from build123d import *

# Parameters (mm, degrees)
EXTRUDE_1_DEPTH     = 3
SKETCH_2_R          = 1.7
SKETCH_2_R_2        = 1.57
CUT_EXTRUDE_1_DEPTH = 3
SKETCH_3_W          = 60
SKETCH_3_H          = 3
EXTRUDE_2_DEPTH     = 5
SKETCH_6_W          = 155
SKETCH_6_H          = 3
EXTRUDE_3_DEPTH     = 4
SKETCH_7_W          = 155
SKETCH_7_H          = 3
EXTRUDE_4_DEPTH     = 4
FILLET_1_R          = 10
CUT_EXTRUDE_3_DEPTH = 4
FILLET_3_R          = 2


with BuildPart() as part:
    # 草图1 → 凸台-拉伸1 (new body)
    with BuildSketch(Plane(origin=(0, 0, 0), x_dir=(1, 0, 0), z_dir=(0, 1, 0))):
        Polygon((0, 0), (7.8, 0), (7.8, 5), (6.1, 5), (6.1, 8), (7.8, 8), (7.8, 13), (11.2, 13), (11.2, 8), (12.9, 8), (12.9, 5), (11.2, 5), (11.2, 0), (17, 0), (17, -3), (25, -3), (25, 0), (31.7, 0), (35, 0), (35, -3), (43, -3), (43, 0), (48.8, 0), (48.8, 5), (47.1, 5), (47.1, 8), (48.8, 8), (48.8, 13), (52.2, 13), (52.2, 8), (53.9, 8), (53.9, 5), (52.2, 5), (52.2, 0), (60, 0), (60, 150), (0, 150), align=None)
    extrude(amount=EXTRUDE_1_DEPTH)

    # 草图2 → 切除-拉伸1 (cut)
    with BuildSketch(Plane(origin=(0, 3, 0), x_dir=(1, 0, 0), z_dir=(0, 1, 0))):
        with Locations(Location((18, 130, 0), (0, 0, 270))):
            Circle(SKETCH_2_R)
        with Locations(Location((42, 130, 0), (0, 0, 270))):
            Circle(SKETCH_2_R_2)
        with Locations(Location((18, 147.9, 0), (0, 0, 270))):
            Circle(SKETCH_2_R)
        with Locations(Location((42, 147.9, 0), (0, 0, 270))):
            Circle(SKETCH_2_R)
        with Locations(Location((42, 31.5, 0), (0, 0, 90))):
            Circle(SKETCH_2_R)
        with Locations(Location((18, 31.5, 0), (0, 0, 90))):
            Circle(SKETCH_2_R)
        with Locations(Location((42, 49.4, 0), (0, 0, 90))):
            Circle(SKETCH_2_R_2)
        with Locations(Location((18, 49.4, 0), (0, 0, 90))):
            Circle(SKETCH_2_R)
        with BuildLine():
            Line((5, 131.7), (10, 131.7))
            ThreePointArc((10, 131.7), (11.7, 130), (10, 128.3))
            Line((10, 128.3), (5, 128.3))
            ThreePointArc((5, 128.3), (3.3, 130), (5, 131.7))
        make_face()
        with BuildLine():
            Line((26, 131.7), (34, 131.7))
            ThreePointArc((34, 131.7), (35.7, 130), (34, 128.3))
            Line((34, 128.3), (26, 128.3))
            ThreePointArc((26, 128.3), (24.3, 130), (26, 131.7))
        make_face()
        with BuildLine():
            Line((50, 131.7), (55, 131.7))
            ThreePointArc((55, 131.7), (56.7, 130), (55, 128.3))
            Line((55, 128.3), (50, 128.3))
            ThreePointArc((50, 128.3), (48.3, 130), (50, 131.7))
        make_face()
        with BuildLine():
            Line((5, 149.6), (10, 149.6))
            ThreePointArc((10, 149.6), (11.7, 147.9), (10, 146.2))
            Line((10, 146.2), (5, 146.2))
            ThreePointArc((5, 146.2), (3.3, 147.9), (5, 149.6))
        make_face()
        with BuildLine():
            Line((26, 149.6), (34, 149.6))
            ThreePointArc((34, 149.6), (35.7, 147.9), (34, 146.2))
            Line((34, 146.2), (26, 146.2))
            ThreePointArc((26, 146.2), (24.3, 147.9), (26, 149.6))
        make_face()
        with BuildLine():
            Line((50, 149.6), (55, 149.6))
            ThreePointArc((55, 149.6), (56.7, 147.9), (55, 146.2))
            Line((55, 146.2), (50, 146.2))
            ThreePointArc((50, 146.2), (48.3, 147.9), (50, 149.6))
        make_face()
        with BuildLine():
            Line((5, 47.7), (10, 47.7))
            ThreePointArc((10, 47.7), (11.7, 49.4), (10, 51.1))
            Line((10, 51.1), (5, 51.1))
            ThreePointArc((5, 51.1), (3.3, 49.4), (5, 47.7))
        make_face()
        with BuildLine():
            Line((26, 47.7), (34, 47.7))
            ThreePointArc((34, 47.7), (35.7, 49.4), (34, 51.1))
            Line((34, 51.1), (26, 51.1))
            ThreePointArc((26, 51.1), (24.3, 49.4), (26, 47.7))
        make_face()
        with BuildLine():
            Line((50, 47.7), (55, 47.7))
            ThreePointArc((55, 47.7), (56.7, 49.4), (55, 51.1))
            Line((55, 51.1), (50, 51.1))
            ThreePointArc((50, 51.1), (48.3, 49.4), (50, 47.7))
        make_face()
        with BuildLine():
            Line((5, 29.8), (10, 29.8))
            ThreePointArc((10, 29.8), (11.7, 31.5), (10, 33.2))
            Line((10, 33.2), (5, 33.2))
            ThreePointArc((5, 33.2), (3.3, 31.5), (5, 29.8))
        make_face()
        with BuildLine():
            Line((26, 29.8), (34, 29.8))
            ThreePointArc((34, 29.8), (35.7, 31.5), (34, 33.2))
            Line((34, 33.2), (26, 33.2))
            ThreePointArc((26, 33.2), (24.3, 31.5), (26, 29.8))
        make_face()
        with BuildLine():
            Line((50, 29.8), (55, 29.8))
            ThreePointArc((55, 29.8), (56.7, 31.5), (55, 33.2))
            Line((55, 33.2), (50, 33.2))
            ThreePointArc((50, 33.2), (48.3, 31.5), (50, 29.8))
        make_face()
    extrude(amount=-CUT_EXTRUDE_1_DEPTH, mode=Mode.SUBTRACT)

    # 草图3 → 凸台-拉伸2 (add)
    with BuildSketch(Plane(origin=(0, 0, -150), x_dir=(-1, 0, 0), z_dir=(0, 0, -1))):
        with Locations((-30, 1.5)):
            Rectangle(SKETCH_3_W, SKETCH_3_H)
    extrude(amount=EXTRUDE_2_DEPTH)

    # 草图6 → 凸台-拉伸3 (add)
    with BuildSketch(Plane(origin=(60, 0, 0), x_dir=(0, 0, -1), z_dir=(1, 0, 0))):
        with Locations((77.5, 1.5)):
            Rectangle(SKETCH_6_W, SKETCH_6_H)
    extrude(amount=EXTRUDE_3_DEPTH)

    # 草图7 → 凸台-拉伸4 (add)
    with BuildSketch(Plane.ZY):
        with Locations((-77.5, 1.5)):
            Rectangle(SKETCH_7_W, SKETCH_7_H)
    extrude(amount=EXTRUDE_4_DEPTH)

    # 圆角1
    fillet_1_edges = [part.edges().sort_by_distance(p)[0] for p in [
        (64, 1.5, -155),
        (-4, 1.5, -155),
    ]]
    fillet(fillet_1_edges, radius=FILLET_1_R)

    # 草图9 → 切除-拉伸3 (cut)
    with BuildSketch(Plane(origin=(0, 3, 0), x_dir=(1, 0, 0), z_dir=(0, 1, 0))):
        Polygon((9.322748518, 120.3), (50.677251482, 120.3), (30, 95.845173728), align=None)
        Polygon((4, 114.204826272), (4, 65.095173728), (24.761804328, 89.65), align=None)
        Polygon((9.407301363, 59.1), (50.592698637, 59.1), (30, 83.454826272), align=None)
        Polygon((56, 114.204826272), (56, 65.095173728), (35.238195672, 89.65), align=None)
    extrude(amount=-CUT_EXTRUDE_3_DEPTH, mode=Mode.SUBTRACT)

    # 圆角3
    fillet_3_edges = [part.edges().sort_by_distance(p)[0] for p in [
        (30, 1.5, -83.454826272),
        (50.592698637, 1.5, -59.1),
        (9.407301363, 1.5, -59.1),
        (56, 1.5, -65.095173728),
        (35.238195672, 1.5, -89.65),
        (56, 1.5, -114.204826272),
        (4, 1.5, -114.204826272),
        (24.761804328, 1.5, -89.65),
        (4, 1.5, -65.095173728),
        (50.677251482, 1.5, -120.3),
        (30, 1.5, -95.845173728),
        (9.322748518, 1.5, -120.3),
    ]]
    fillet(fillet_3_edges, radius=FILLET_3_R)


solid = part.part
Verification items for the finished model (mm, model axes). A direction names the side the tool comes from. Coordinates: 2 decimals unless noted, no trailing zeros. Order: outer loops, then holes, each group sorted by start corner. A loop starts at its lowest first (then second) coordinate and runs counter-clockwise, first axis right, second up. Notation, with made-up numbers: M 28.25,-31.5 L 42.25,-31.5 A21 ccw 42.25,-10.5 Z; hole C 4,42 d1. An arc over 180 degrees is marked long. One line per item, written item: value. Start each with the question number.
Item 1: Scan lines: probe 1 along X at (y, z) = (1.45, -49.4); probe 2 along X at (y, z) = (1.8, -31.5); probe 3 along X at (y, z) = (1.45, -76.5). Record each from-to range of solid material in increasing order.
Item 2: Sectioned sample at C-C (x = 60). Enter the section's corners in (y, z).
Item 3: Mould release check, pull along Z, two halves, no side actions. Record for faces 1 (the flat face through (35, 1, 1)), 2 (the cylindrical face through (56.7, 1.5, -49.4)), 3 (the flat face through (2, 1, 0)): released by +Z, released by -Z, zero draft, split by the parting line, or undercut.
Item 4: Sectioned sample at B-B (z = -49.4). Enter the section's corners in (x, y).
Item 5: Sectioned sample at D-D (y = 1.8). Count the separate pieces of the cut face and the enclosed holes in it, then the cut area to 3 significant figures.
Item 6: Sectioned sample at A-A (z = -11). Enter the section's corners in (x, y).
Item 7: Gauge pin test, flat ends, axial feed: pin 1 (0.9 mm diameter, centred on x = 52.5, y = 1.5, fed in from +Z); pin 2 (1.5 mm diameter, centred on x = 56.5, y = 1.5, fed in from -Z); pin 3 (1.5 mm diameter, centred on x = 50.5, y = 1, fed in from +Z). Record the tip position at first contact, or that the pin passes through.
Item 8: Access from +Z, -Z, +X, -X, +Y, -Y to the whole of each face (thin tool, end or side, straight path). Record for faces 4 (the flat face through (7, 2, -29.8)), 5 (the flat face through (7.8, 1, -2)).
Conclusion:
1. probe 1: x = -4 to 3.3, 11.7 to 16.3, 19.7 to 24.3, 35.7 to 40.43, 43.57 to 48.3, 56.7 to 64
1. probe 2: x = -4 to 3.3, 11.7 to 16.3, 19.7 to 24.3, 35.7 to 40.3, 43.7 to 48.3, 56.7 to 64
1. probe 3: x = -4 to 4, 13.64 to 24.12, 35.88 to 46.36, 56 to 64
2. outline: M 0,-153 L 3,-153 L 3,0 L 0,0 Z
3. face 1: zero draft
3. face 2: undercut
3. face 3: released by +Z
4. outline: M -4,0 L 3.3,0 L 3.3,3 L -4,3 Z; M 11.7,0 L 16.3,0 L 16.3,3 L 11.7,3 Z; M 19.7,0 L 24.3,0 L 24.3,3 L 19.7,3 Z; M 35.7,0 L 40.43,0 L 40.43,3 L 35.7,3 Z; M 43.57,0 L 48.3,0 L 48.3,3 L 43.57,3 Z; M 56.7,0 L 64,0 L 64,3 L 56.7,3 Z
5. separate pieces: 1
5. enclosed holes: 24
5. area: 8,030 mm^2
6. outline: M -4,0 L 7.8,0 L 7.8,3 L -4,3 Z; M 11.2,0 L 48.8,0 L 48.8,3 L 11.2,3 Z; M 52.2,0 L 64,0 L 64,3 L 52.2,3 Z
7. pin 1: stops at z = 0
7. pin 2: stops at z = -154.85
7. pin 3: stops at z = -13
8. face 4: +Y, -Y
8. face 5: +Z, +Y, -Y
